Could you check a few things on this model? Use its own coordinates, in mm. Face numbers are marked on the shaded views. A direction names the side the tool comes from. Coordinates: 2 decimals unless noted, no trailing zeros. Loops run counter-clockwise (first coordinate to the right, second up) from the corner with the lowest first, then second, coordinate; pieces in that order, holes last. Notation, with made-up numbers: (54, 1) -> (68, 1) arc R26 cw to (68, 36) -> close; hole circle Ø6 at (52.5, -31.75). An arc over 180 degrees is marked (long way). One line per question, with ' | ' between items.
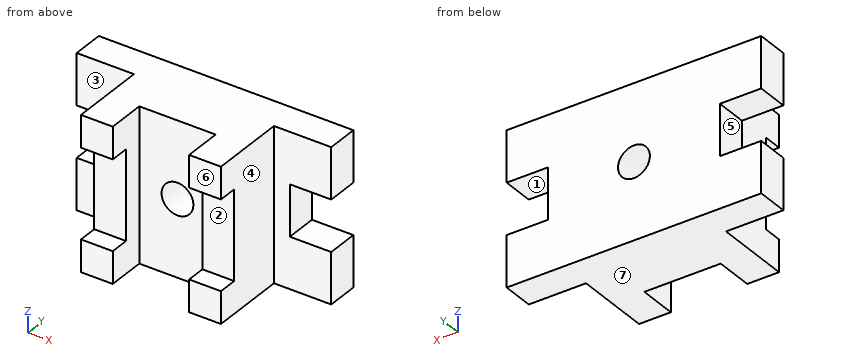
from build123d import *

# Parameters (mm, degrees)
F1_DEPTH  = 31.75
F2_W      = 139.7
F2_H      = 152.4
F3_DEPTH  = 38.1
F4_W      = 31.75
F4_H      = 152.4
F5_DEPTH  = 19.05
F4_R      = 15.875
F6_DEPTH  = 69.851
F7_W      = 31.75
F7_H      = 31.75
F8_DEPTH  = 19.05
F9_W      = 31.75
F9_H      = 31.75
F10_DEPTH = 19.05


with BuildPart() as f1:
    # F0 (on Front) → F1 (new body)
    with BuildSketch(Plane.XZ):
        Polygon((179.5150149531, 50.8), (-74.4849850469, 50.8), (-74.4849850469, 0), (-33.2099850469, 0), (-33.2099850469, -50.8), (-74.4849850469, -50.8), (-74.4849850469, -101.6), (179.5150149531, -101.6), (179.5150149531, -50.8), (138.2400149531, -50.8), (138.2400149531, 0), (179.5150149531, 0), align=None)
    extrude(amount=F1_DEPTH)

    # F2 (on face) → F3 (join)
    with BuildSketch(Plane.XZ.offset(31.75)):
        with Locations((52.5150149531, -25.4)):
            Rectangle(F2_W, F2_H)
    extrude(amount=F3_DEPTH)

    # F4 (on face) → F5 (join)
    with BuildSketch(Plane.XZ.offset(69.85)):
        with Locations((-1.4599850469, -25.4)):
            Rectangle(F4_W, F4_H)
        with Locations((106.4900149531, -25.4)):
            Rectangle(F4_W, F4_H)
    extrude(amount=F5_DEPTH)

    # F4 (on face) → F6 (cut, through all)
    with BuildSketch(Plane.XZ.offset(69.85)):
        with Locations((52.5150149531, -25.4)):
            Circle(F4_R)
    extrude(amount=-F6_DEPTH, mode=Mode.SUBTRACT)

    # F7 (on face) → F8 (join)
    with BuildSketch(Plane.XZ.offset(88.9)):
        with Locations((-1.4599850469, 34.925)):
            Rectangle(F7_W, F7_H)
        with Locations((-1.4599850469, -85.725)):
            Rectangle(F7_W, F7_H)
    extrude(amount=F8_DEPTH)

    # F9 (on face) → F10 (join)
    with BuildSketch(Plane.XZ.offset(88.9)):
        with Locations((106.4900149531, 34.925)):
            Rectangle(F9_W, F9_H)
        with Locations((106.4900149531, -85.725)):
            Rectangle(F9_W, F9_H)
    extrude(amount=F10_DEPTH)


solid = f1.part
1) I'm going to push flat-ended pins straight in: pin 1 Ø6 at (y, z) = (-15, -33) entering from +X; pin 2 Ø4 at (x, y) = (74.5, -73) entering from +Z; pin 3 Ø1 at (y, z) = (-62, -9.5) entering from +X (3 decimals); pin 4 Ø12 at (x, z) = (61.5, -15.5) entering from +Y. Where does each tip first touch, or does it pass through?
Data:
pin 1: x = 138.24 | pin 2: through | pin 3: x = 122.365 | pin 4: y = 0
2) If we section it at D-D on z = 41: Please give me the cut outline in (x, y), and give its area (3 significant figures).
Data:
outline: (-74.48, -31.75) -> (-17.33, -31.75) -> (-17.33, -107.95) -> (14.42, -107.95) -> (14.42, -69.85) -> (90.62, -69.85) -> (90.62, -107.95) -> (122.37, -107.95) -> (122.37, -31.75) -> (179.52, -31.75) -> (179.52, 0) -> (-74.48, 0) -> close | area: 15,800 mm²
3) I need wall thicknesses on line 1 along X through (y, z) = (-78, -31.5); line 2 along Z through (x, y) = (160.5, -27.5); line 3 along X through (y, z) = (-18, -25). Which ranges of each line are inside material? Lowest first, please. Write a range as from..to.
Data:
line 1: -17.33..14.42, 90.62..122.37 | line 2: -101.6..-50.8, 0..50.8 | line 3: -33.21..36.65, 68.38..138.24
4) If we section it at C-C on y = -95.5: Please give me the cut outline in (x, z), and give its area (3 significant figures).
Data:
outline: (-17.33, -101.6) -> (14.42, -101.6) -> (14.42, -69.85) -> (-17.33, -69.85) -> close; (-17.33, 19.05) -> (14.42, 19.05) -> (14.42, 50.8) -> (-17.33, 50.8) -> close; (90.62, -101.6) -> (122.37, -101.6) -> (122.37, -69.85) -> (90.62, -69.85) -> close; (90.62, 19.05) -> (122.37, 19.05) -> (122.37, 50.8) -> (90.62, 50.8) -> close | area: 4,030 mm²
5) On a 3-axis mill with a long thin cutter (end or side, diameter ignored), from which of +Z, -Z, +X, -X, +Y, -Y can I reach the whole of each face in a straight line? I mean the marked faces 1, 2, 3 and 4. Say none if no direction works.
Data:
face 1: +X, +Y, -Y | face 2: +X, -X, -Y | face 3: +Z, -Z, -X, -Y | face 4: +Z, -Z, +X, -Y
6) We'd pull the mould along Z, two halves only. Please class the marked faces 5, 6 and 7: pulls with the +Z half, pulls with the -Z half, needs draft (parallel to the pull), parting line crosses it, or undercut.
Data:
face 5: undercut | face 6: needs draft | face 7: pulls with the -Z half
7) If we section it at B-B on z = -25.4: Please give me the cut outline in (x, y), and give its area (3 significant figures).
Data:
outline: (-33.21, -31.75) -> (-17.33, -31.75) -> (-17.33, -88.9) -> (14.42, -88.9) -> (14.42, -69.85) -> (36.64, -69.85) -> (36.64, 0) -> (-33.21, 0) -> close; (68.39, -69.85) -> (90.62, -69.85) -> (90.62, -88.9) -> (122.37, -88.9) -> (122.37, -31.75) -> (138.24, -31.75) -> (138.24, 0) -> (68.39, 0) -> close | area: 9,760 mm²
8) If we section it at A-A on y = -74: Please give me the cut outline in (x, z).
Data:
outline: (-17.33, -101.6) -> (14.42, -101.6) -> (14.42, 50.8) -> (-17.33, 50.8) -> close; (90.62, -101.6) -> (122.37, -101.6) -> (122.37, 50.8) -> (90.62, 50.8) -> close
